Could you check a few things on this model? Use its own coordinates, in mm. Face numbers are marked on the shaded views. A direction names the side the tool comes from. Round coordinates to 2 decimals unless told otherwise and drop trailing zeros. Loops run counter-clockwise (first coordinate to the right, second up) from the corner with the lowest first, then second, coordinate; pieces in that order, holes last. Notation, with made-up numbers: (31.25, 24) -> (81.25, 24) arc R17 ccw to (81.25, 52) -> close; hole circle Ø1 at (78.5, -5). An arc over 180 degrees is marked (long way). Put each result on its own line as item: value. Start each with the question number.
1. Imagine slicing it at A-A, the plane z = 10. Please give me the cut outline in (x, y).
2. Imagine slicing it at C-C, the plane x = 7. Please give me the cut outline in (y, z), and give its area (3 significant figures).
3. I'm going to push flat-ended pins straight in: P1, Ø3, axis at x = 16.5, z = 9, coming from the +Y side; P2, Ø1.5, axis at x = 4, z = 2.5, coming from the +Y side; P3, Ø5.5, axis at x = 7.5, z = 12, coming from the +Y side. Where does each tip first touch, or does it pass through?
4. Which directions (+Z, -Z, +X, -X, +Y, -Y) give clear straight access to the entire face, cutting with the end or side of a thin tool? Please do the marked faces 4, 5 and 6.
5. Imagine slicing it at D-D, the plane x = 14. Please give me the cut outline in (y, z), and give its area (3 significant figures).
6. Imagine slicing it at B-B, the plane z = 17.75. Please give me the cut outline in (x, y).
7. I need wall thicknesses on line 1 (Z direction, x = 5, y = 10); line 2 (X direction, y = 16.5, z = 12); line 3 (X direction, y = 11, z = 18.25). Which ranges of each line are inside material? Lowest first, please. Write a range as [from, to].
8. If we mould it in two halves opening along Z, with no side actions, what happens to the marked faces 1, 2 and 3? For each: pulls with the +Z half, pulls with the -Z half, needs draft (parallel to the pull), parting line crosses it, or undercut.
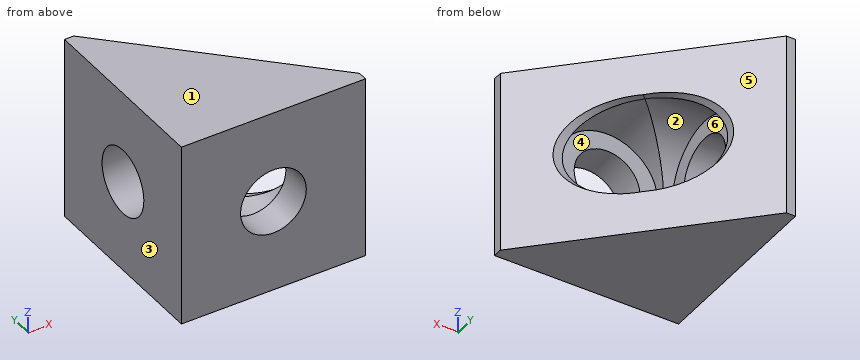
Autodesk Inventor part; units mm, degrees
ref_plane "Work Plane1" through (20, 1.0001, 20) normal (-1, 0, 0) x (0, 0, 1)
ref_plane "YZ Plane" through (0, 0, 0) normal (1, 0, 0) x (0, 1, 0)
ref_plane "XZ Plane" through (0, 0, 0) normal (0, 1, 0) x (-1, 0, 0)
sketch "Sketch1" plane through (0, 0, 0) normal (0, 0, 1) x (1, 0, 0)
  line L0 (0, 0) -> (0, 20)
  line L1 (20, 0) -> (0, 0)
  line L2 (0, 20) -> (1, 20)
  line L3 (1, 20) -> (20, 1.0001)
  line L4 (20, 1.0001) -> (20, 0)
  dimension "d0" = 20
  dimension "d1" = 20
  dimension "d2" = 1
  dimension "d3" = 26.87
  dimension "d4" = 1.0001
extrude "Extrusion1" add sketch "Sketch1" along normal blind 20
sketch "Sketch2" plane through (0, 0, 0) normal (-1, 0, 0) x (0, 0, 1)
  line L0 (0, 0) -> (20, 0)
  circle A0 centre (10, 10) radius 3.57
  circle A1 centre (10, 10) radius 5.5
  line L1 (10, 19.6278) -> (10, 0) construction
  dimension "d7" = 7.14
  dimension "d8" = 11
  dimension "d9" = 4.5
extrude "Extrusion2" cut sketch "Sketch2" against normal through all contours A0
sketch "Sketch3" plane through (0, 0, 0) normal (0, -1, 0) x (1, 0, 0)
  circle A0 centre (10, 10) radius 3.57
  dimension "d12" = 7.14
extrude "Extrusion3" cut sketch "Sketch3" against normal through all
ref_plane "Work Plane1" through (20, 1.0001, 20) normal (-1, 0, 0) x (0, 0, 1)
sketch "Sketch4" plane through (20, 1.0001, 20) normal (-1, 0, 0) x (0, 0, 1)
  circle A0 centre (-10, 8.9999) radius 3.57
  circle A1 centre (-10, 8.9999) radius 5.5
  point P0 (-20, -1.0001)
  dimension "d15" = 11
extrude "Extrusion4" cut sketch "Sketch4" along normal blind 16.5
sketch "Sketch5" plane through (0, 20, 0) normal (0, 1, 0) x (1, 0, 0)
  circle A0 centre (10, -10) radius 5.5
  dimension "d18" = 11
extrude "Extrusion5" cut sketch "Sketch5" against normal blind 16.5
equation "\"d1\" = d0"
properties part number "90 Degree Corner Connector" material "Acetal Resin, White"
Entries:
1. outline: (0, 0) -> (6.43, 0) -> (6.43, 3.5) -> (4.5, 3.5) -> (4.5, 4.5) -> (3.5, 4.5) -> (3.5, 6.43) -> (0, 6.43) -> close; (0, 13.57) -> (3.5, 13.57) -> (3.5, 15.5) -> (4.5, 15.5) -> (4.5, 16.5) -> (1, 20) -> (0, 20) -> close; (13.57, 0) -> (20, 0) -> (20, 1) -> (16.5, 4.5) -> (15.5, 4.5) -> (15.5, 3.5) -> (13.57, 3.5) -> close
2. outline: (0, 0) -> (14, 0) -> (14, 5.39) -> (13, 5.39) arc R5.5 cw to (7, 5.39) -> (3.5, 5.39) -> (3.5, 8.06) -> (0, 8.06) -> close; (0, 11.94) -> (3.5, 11.94) -> (3.5, 14.61) -> (7, 14.61) arc R5.5 cw to (13, 14.61) -> (14, 14.61) -> (14, 20) -> (0, 20) -> close
2. area: 162 mm^2
3. P1: y = 5.05
3. P2: y = 17.75
3. P3: y = 16.25
4. face 4: +Y
4. face 5: +Z, -Z, +X, +Y
4. face 6: +X
5. outline: (0, 0) -> (7, 0) -> (7, 5.39) arc R5.5 cw to (6, 6.23) -> (3.5, 6.23) -> (3.5, 13.77) -> (6, 13.77) arc R5.5 cw to (7, 14.61) -> (7, 20) -> (0, 20) -> close
5. area: 113 mm^2
6. outline: (0, 0) -> (20, 0) -> (20, 1) -> (1, 20) -> (0, 20) -> close
7. line 1: [0, 4.5], [15.5, 20]
7. line 2: [0, 4.5]
7. line 3: [0, 10]
8. face 1: pulls with the +Z half
8. face 2: undercut
8. face 3: needs draft
